from build123d import *

# Parameters (mm, degrees)
PAD_DEPTH       = 2
PAD001_DEPTH    = 13
SKETCH002_W     = 10
SKETCH002_H     = 15
PAD002_DEPTH    = 3
SKETCH003_R     = 1.7
POCKET_DEPTH    = 27.001
SKETCH004_R     = 1.7
POCKET001_DEPTH = 15.001


with BuildPart() as part:
    # Sketch → Pad (new body)
    with BuildSketch(Plane.XY):
        Polygon((-12, 15), (-12, -14), (15, -14), (15, 0), (0, 0), (0, 15), align=None)
    extrude(amount=PAD_DEPTH)

    # Sketch001 → Pad001 (new body)
    with BuildSketch(Plane(origin=(0, 0, 0), x_dir=(1, 0, 0), z_dir=(0, 0, -1))):
        Polygon((-12, -15), (-12, 14), (15, 14), (15, 12), (-10, 12), (-10, -15), align=None)
    extrude(amount=PAD001_DEPTH)

    # Sketch002 → Pad002 (new body)
    with BuildSketch(Plane(origin=(0, 0, 0), x_dir=(1, 0, 0), z_dir=(0, 0, -1))):
        with Locations((-5, -7.5)):
            Rectangle(SKETCH002_W, SKETCH002_H)
    extrude(amount=PAD002_DEPTH)

    # Sketch003 → Pocket (cut, through all)
    with BuildSketch(Plane(origin=(-12, 0, 0), x_dir=(0, -1, 0), z_dir=(-1, 0, 0))):
        with Locations((-7.5, -8)):
            Circle(SKETCH003_R)
        with Locations((6, -8)):
            Circle(SKETCH003_R)
    extrude(amount=-POCKET_DEPTH, mode=Mode.SUBTRACT)

    # Sketch004 → Pocket001 (cut, through all)
    with BuildSketch(Plane.XY.offset(2)):
        with Locations((-4, -6)):
            Circle(SKETCH004_R)
    extrude(amount=-POCKET001_DEPTH, mode=Mode.SUBTRACT)


solid = part.part
Design review of the part built by this model. Coordinates are the model's own, in mm. A direction names the side the tool comes from. Give positions to 0.01 mm unless a question says otherwise; leave off trailing zeros. Write each loop counter-clockwise with the first axis right and the second up, starting at its lowest first coordinate (ties: lowest second). Pieces come first, ordered by that corner, then holes. Notation, with made-up numbers: M 18.25,57 L 59.25,57 A29 cw 59.25,79 Z; hole C 77.25,-28.5 d9. An arc over 180 degrees is marked long. Answer as a JSON object with one key per item and string values. Group by question number.
1) We need section D-D (z = -8). Give the boundary of the cut face in (x, y), and give its area (3 significant figures).
2) Tool access review of faces 4 (the face through (-5, 7, -3)), 5 (the face through (-12, 1, -5)), 6 (the face through (-5, 0, -1)), 7 (the face through (8, 0, 1)), 8 (the face through (-11.01, -5.63, -9.66)): name each direction out of +Z, -Z, +X, -X, +Y, -Y from which nothing blocks a thin tool from reaching the whole face with its end or side.
3) Mouldability with a two-part tool opening along Y and no side actions: class faces 1 (the face through (-11.01, 7.87, -9.66)), 2 (the face through (1, -14, -5)), 3 (the face through (0, 8, 0)) as released by +Y, released by -Y, zero draft, split by the parting line, or undercut.
4) We need section A-A (y = -6). Give the boundary of the cut face in (x, z).
5) We need section B-B (y = 7.5). Give the boundary of the cut face in (x, z).
6) We need section C-C (x = -4). Give the boundary of the cut face in (y, z), and give its area (3 significant figures).
7) For line 1 along Y through (x, z) = (-4, 1.6); line 2 along Z through (x, y) = (-10.35, 7.5); line 3 along X through (y, z) = (8.5, -4.5), list the stretches that pass through material, from the lowest coordinate up.
8) Clearance check with flat-ended pins moving along their axes: pin 1 Ø6 at (y, z) = (11, 0) entering from +X; pin 2 Ø4.5 at (y, z) = (7.5, -8) entering from +X; pin 3 Ø4 at (x, z) = (7.5, -7.5) entering from +Y. State where each tip first meets the part, or that it passes through.
Answer key:
{
 "1": {"outline": "M -12,-14 L 15,-14 L 15,-12 L -10,-12 L -10,-7.7 L -12,-7.7 Z; M -12,-4.3 L -10,-4.3 L -10,5.8 L -12,5.8 Z; M -12,9.2 L -10,9.2 L -10,15 L -12,15 Z", "area": "94.4 mm²"},
 "2": {"face 4": "-Z, +X, +Y", "face 5": "+Z, -Z, -X, +Y, -Y", "face 6": "-Z, +X", "face 7": "+Z, -Z, +X, +Y", "face 8": "+X, -X"},
 "3": {"face 1": "undercut", "face 2": "released by -Y", "face 3": "zero draft"},
 "4": {"outline": "M -12,-13 L -10,-13 L -10,-9.7 L -12,-9.7 Z; M -12,-6.3 L -10,-6.3 L -10,0 L -5.7,0 L -5.7,2 L -12,2 Z; M -2.3,0 L 15,0 L 15,2 L -2.3,2 Z"},
 "5": {"outline": "M -12,-13 L -10,-13 L -10,-9.7 L -12,-9.7 Z; M -12,-6.3 L -10,-6.3 L -10,-3 L 0,-3 L 0,2 L -12,2 Z"},
 "6": {"outline": "M -14,-13 L -12,-13 L -12,0 L -7.7,0 L -7.7,2 L -14,2 Z; M -4.3,0 L 0,0 L 0,-3 L 15,-3 L 15,2 L -4.3,2 Z", "area": "122 mm²"},
 "7": {"line 1": "y = -14 to -7.7, -4.3 to 15", "line 2": "z = -13 to -9.7, -6.3 to 2", "line 3": "x = -12 to -10"},
 "8": {"pin 1": "stops at x = 0", "pin 2": "stops at x = -10", "pin 3": "stops at y = -12"}
}
